```python
from build123d import *

# Parameters (mm, degrees)
EXTRUDE_1_DEPTH        = 28
FILLET_1_R             = 1
SWEEP_1_PROFILE_R      = 0.7
PATTERN_LINEAR_1_COUNT = 2
PATTERN_LINEAR_1_PITCH = 2.5


with BuildPart() as part:
    # 草图1 → 凸台-拉伸1 (new body)
    with BuildSketch(Plane(origin=(0, 0, 0), x_dir=(0, 0, -1), z_dir=(1, 0, 0))):
        Polygon((0, 0), (0, 31), (2, 31), (5.7, 24), (5.7, 0), align=None)
    extrude(amount=EXTRUDE_1_DEPTH)

    # 圆角1
    fillet_1_edges = [part.edges().sort_by_distance(p)[0] for p in [
        (28, 27.5, -3.85),
        (28, 31, -1),
        (28, 15.5, 0),
        (28, 0, -2.85),
        (0, 15.5, 0),
        (0, 31, -1),
        (0, 27.5, -3.85),
        (0, 12, -5.7),
        (0, 0, -2.85),
        (28, 12, -5.7),
        (14, 0, 0),
        (14, 31, 0),
        (14, 31, -2),
        (14, 24, -5.7),
        (14, 0, -5.7),
    ]]
    fillet(fillet_1_edges, radius=FILLET_1_R)

    # 扫描1: sweep along a path in 草图2
    with BuildLine(Plane.XY.offset(-1.3)) as sweep_1_path:
        ThreePointArc((4.001651966, 34.019317003), (2.935743371, 31.239649146), (4.579965561, 28.757865933))
    # 扫描1 profile (on start of the path) → 扫描1 (sweep)
    with BuildSketch(Plane(origin=(4.001651966, 34.019317003, -1.3), x_dir=(0.6661061501000685, -0.745856954649392, 0), z_dir=(-0.745856954649392, -0.6661061501000685, 0))):
        Circle(SWEEP_1_PROFILE_R)
    sweep_1 = sweep(path=sweep_1_path.line)

    # 阵列(线性)1: 扫描1 ×2
    with Locations(*[(i * PATTERN_LINEAR_1_PITCH, 0, 0) for i in range(1, PATTERN_LINEAR_1_COUNT)]):
        add(sweep_1)


solid = part.part
```
Design review of the part built by this model. Coordinates are the model's own, in mm. Coordinates: 2 decimals unless noted, no trailing zeros. Order: outer loops, then holes, each group sorted by start corner. A loop starts at its lowest first (then second) coordinate and runs counter-clockwise, first axis right, second up. Notation, with made-up numbers: (14, 38) - (30, 38) arc R13 cw to (30, 56) - close; hole circle Ø1 at (76.5, 28). An arc over 180 degrees is marked (long way). One line per question, with ' | ' between items.
Q1. Clearance check with a flat-ended pin moving along its axis: pin 1 Ø2 at (x, y) = (3.5, 28) entering from -Z. State where the tip first meets the part, or that it passes through.
Answer key:
pin 1: stops at z = -4.11
Q2. To check wall thickness, follow line 1 along Y through (x, z) = (13, -1.15); line 2 along Y through (x, z) = (1.5, -1.8); line 3 along X through (y, z) = (25, -0.85). State the ranges of each line that lie inside material, in increasing order.
Answer key:
line 1: y = 0 to 31 | line 2: y = 0 to 30.92 | line 3: x = 0.01 to 27.99
Q3. Consider section A-A, the plane x = 15.5. Give the boundary of the cut face in (y, z), then the cut area to 3 significant figures.
Answer key:
outline: (0, -4.7) arc R1 ccw to (1, -5.7) - (23.75, -5.7) arc R1 ccw to (24.22, -5.58) - (30.47, -2.28) arc R1 ccw to (31, -1.4) - (31, -1) arc R1 ccw to (30, 0) - (1, 0) arc R1 ccw to (0, -1) - close | area: 163 mm2
